```python
from build123d import *

# Parameters (mm, degrees)
BOSS_EXTRU_1_DEPTH = 6
CONG_1_R           = 1000
CONG_2_R           = 500
CONG_4_R           = 10
CONG_5_R           = 5
CONG_6_R           = 500


with BuildPart() as part:
    # Esquisse2 → Boss.-Extru.1 (new body)
    with BuildSketch(Plane.XY):
        Polygon((0, 0), (-800, 0), (-963.993473565, 96.541430402), (-1163.117471936, 180.636697165), (-1032.508966499, 163.110428865), (-1032.508966499, 141.610428865), (-1029.508966499, 141.610428865), (-1029.508966499, 162.707860864), (-980.08668451, 156.075917781), (-854.092873153, 81.904534581), (-854.092873153, 60.404534581), (-851.092873153, 60.404534581), (-851.092873153, 80.138462524), (-799.897120857, 50), (-637.333486788, 50), (-637.333486788, 28.5), (-634.333486788, 28.5), (-634.333486788, 50), (-252.546237876, 50), (-252.546237876, 28.5), (-249.546237876, 28.5), (-249.546237876, 50), (-157.380204695, 50), (-42.620023216, 164.760181479), (-3, 164.760181479), (-3, 130.978409526), (0, 130.978409526), (0, 115.978409526), (-60.96795982, 55.010449706), (-60.96795982, 15.54862942), (0, 15.54862942), align=None)
    extrude(amount=BOSS_EXTRU_1_DEPTH)

    # Congé1
    cong_1_edges = [part.edges().sort_by_distance(p)[0] for p in [
        (-963.993473565, 96.541430402, 3),
    ]]
    fillet(cong_1_edges, radius=CONG_1_R)

    # Congé2
    cong_2_edges = [part.edges().sort_by_distance(p)[0] for p in [
        (-800, 0, 3),
    ]]
    fillet(cong_2_edges, radius=CONG_2_R)

    # Congé4
    cong_4_edges = [part.edges().sort_by_distance(p)[0] for p in [
        (0, 0, 3),
    ]]
    fillet(cong_4_edges, radius=CONG_4_R)

    # Congé5
    cong_5_edges = [part.edges().sort_by_distance(p)[0] for p in [
        (-1163.117471936, 180.636697165, 3),
    ]]
    fillet(cong_5_edges, radius=CONG_5_R)

    # Congé6
    # the kernel refuses this fillet: 500 mm, written as the material it adds along each edge
    with BuildSketch(Plane(origin=(-799.897120857, 50, 0), x_dir=(-0.8617626627439038, 0.5073116528333809, 0), z_dir=(0, 0, 1))) as cong_6_piece_1_section:
        with BuildLine():
            CenterArc((150.440377281, -491.643304898), CONG_6_R, 100.490027974, 19.994897644)
            Line((-103.215449136, -60.761973526), (-108.288565664, -52.144346898))
            Line((-108.288565664, -52.144346898), (-5.073116528, 8.617626627))
            Line((-5.073116528, 8.617626627), (0, 10))
            ThreePointArc((0, 10), (29.704090529, 10), (57.587537133, 9.832866098))
            Line((57.587537133, 9.832866098), (59.408181057, 0))
        make_face()
    cong_6_piece_1 = extrude(amount=6, mode=Mode.PRIVATE)
    cong_6_piece_1 = split(cong_6_piece_1, bisect_by=Plane(origin=(-851.092873153, 52.596718386, 3), z_dir=(1, 0, 0)), keep=Keep.TOP, mode=Mode.PRIVATE)
    add(cong_6_piece_1)


solid = part.part
```
Model file for the job. Use its own axes, mm. A direction names the side the tool comes from. Give positions to 0.01 mm unless a question says otherwise; leave off trailing zeros. Loops run counter-clockwise (first coordinate to the right, second up) from the corner with the lowest first, then second, coordinate; pieces in that order, holes last. Notation, with made-up numbers: (-26.75, 15) -> (-13.75, 15) arc R15 ccw to (-13.75, 34) -> close; hole circle Ø8 at (7, 3.25). An arc over 180 degrees is marked (long way). Write each question's results on one line, items separated by ' | '.
(1) Pull direction Y, two halves, no side cores. Call faces 3 (the cylindrical face through (-768.1, 57.8, 3)), 4 (the flat face through (-466, 32, 6)), 5 (the flat face through (-30.06, 85.92, 2.96)): released by +Y, released by -Y, zero draft, split by the parting line, or undercut.
Geometry results:
face 3: released by +Y | face 4: zero draft | face 5: undercut
(2) Tool access for faces 1 (the flat face through (-100.8, 106.58, 2.96)), 2 (the cylindrical face through (-967.886, 96.033, 3.042)): list every direction of +Z, -Z, +X, -X, +Y, -Y with a clear straight run to the whole face (end or side of a thin tool).
Geometry results:
face 1: +Z, -Z, +Y | face 2: +Z, -Z, -X, -Y
(3) Cut at B-B on x = -343. List the corners of the cut face in (y, z).
Geometry results:
outline: (0, 0) -> (50, 0) -> (50, 6) -> (0, 6) -> close
(4) Cut at C-C on x = -1000.5. List the corners of the cut face in (y, z).
Geometry results:
outline: (111.57, 0) -> (158.82, 0) -> (158.82, 6) -> (111.57, 6) -> close
(5) Probe line 1 along X through (y, z) = (40, 5.5); line 2 along Y through (x, z) = (-525.5, 5.5); line 3 along X through (y, z) = (140, 2.5). List the from-to ranges inside material, lowest first.
Geometry results:
line 1: x = -859.81 to -637.33, -634.33 to -252.55, -249.55 to -60.97 | line 2: y = 0 to 50 | line 3: x = -1066.9 to -952.78, -67.38 to -3
(6) Cut at A-A on y = 92. List the corners of the cut face in (x, z), and give its area (3 significant figures).
Geometry results:
outline: (-959.89, 0) -> (-871.24, 0) -> (-871.24, 6) -> (-959.89, 6) -> close; (-115.38, 0) -> (-23.98, 0) -> (-23.98, 6) -> (-115.38, 6) -> close | area: 1,080 mm²
(7) Flat gauge pins, fed straight in: pin 1 Ø1.8 at (y, z) = (36.5, 1.5) entering from -X; pin 2 Ø0.9 at (x, z) = (-251, 2) entering from +Y; pin 3 Ø2.5 at (x, z) = (-635, 4) entering from +Y. Where does each tip first touch, or does it go through?
Geometry results:
pin 1: stops at x = -853.6 | pin 2: stops at y = 28.5 | pin 3: stops at y = 50
